```python
from build123d import *

# Parameters (mm, degrees)
SKETCH2_R           = 7.25
SKETCH2_R_2         = 2.25
SKETCH2_W           = 22
SKETCH2_H           = 44
BOSS_EXTRUDE1_DEPTH = 6
CUT_EXTRUDE1_START  = -26
CUT_EXTRUDE1_DEPTH  = 26


with BuildPart() as part:
    # Sketch2 → Boss-Extrude1 (new body)
    with BuildSketch(Plane(origin=(0, 0, 0), x_dir=(1, 0, 0), z_dir=(0, 1, 0))):
        with BuildLine():
            Line((-16.25, 90), (-16.25, -90))
            ThreePointArc((-16.25, -90), (0, -106.25), (16.25, -90))
            Line((16.25, -90), (16.25, 90))
            ThreePointArc((16.25, 90), (0, 106.25), (-16.25, 90))
        make_face()
        with Locations(Location((0, 90, 0), (0, 0, 270))):
            Circle(SKETCH2_R, mode=Mode.SUBTRACT)
        with Locations(Location((0, -90, 0), (0, 0, 270))):
            Circle(SKETCH2_R, mode=Mode.SUBTRACT)
        with Locations(Location((8, 98, 0), (0, 0, 270))):
            Circle(SKETCH2_R_2, mode=Mode.SUBTRACT)
        with Locations(Location((-8, 98, 0), (0, 0, 270))):
            Circle(SKETCH2_R_2, mode=Mode.SUBTRACT)
        with Locations(Location((-8, 82, 0), (0, 0, 270))):
            Circle(SKETCH2_R_2, mode=Mode.SUBTRACT)
        with Locations(Location((8, 82, 0), (0, 0, 270))):
            Circle(SKETCH2_R_2, mode=Mode.SUBTRACT)
        with Locations(Location((8, -98, 0), (0, 0, 90))):
            Circle(SKETCH2_R_2, mode=Mode.SUBTRACT)
        with Locations(Location((8, -82, 0), (0, 0, 90))):
            Circle(SKETCH2_R_2, mode=Mode.SUBTRACT)
        with Locations(Location((-8, -82, 0), (0, 0, 90))):
            Circle(SKETCH2_R_2, mode=Mode.SUBTRACT)
        with Locations(Location((-8, -98, 0), (0, 0, 90))):
            Circle(SKETCH2_R_2, mode=Mode.SUBTRACT)
        with Locations(Location((-5, 63.652785483, 0), (0, 0, 270))):
            Circle(SKETCH2_R_2, mode=Mode.SUBTRACT)
        with Locations(Location((5, 63.652785483, 0), (0, 0, 270))):
            Circle(SKETCH2_R_2, mode=Mode.SUBTRACT)
        with Locations(Location((-5, 14.152785483, 0), (0, 0, 270))):
            Circle(SKETCH2_R_2, mode=Mode.SUBTRACT)
        with Locations(Location((5, 14.152785483, 0), (0, 0, 270))):
            Circle(SKETCH2_R_2, mode=Mode.SUBTRACT)
        with Locations(Location((0, -36.453, 0), (0, 0, 270))):
            Circle(SKETCH2_R_2, mode=Mode.SUBTRACT)
        with Locations((0, 38.902785483)):
            Rectangle(SKETCH2_W, SKETCH2_H, mode=Mode.SUBTRACT)
    extrude(amount=BOSS_EXTRUDE1_DEPTH)

    # Sketch3 → Cut-Extrude1 (cut)
    with BuildSketch(Plane(origin=(0, 6, 0), x_dir=(1, 0, 0), z_dir=(0, 1, 0)).offset(CUT_EXTRUDE1_START)):
        with BuildLine():
            ThreePointArc((-2, -31.59887804), (-3.249097876, -32.329183443), (-4.25140088, -33.372725571))
            Line((-4.25140088, -33.372725571), (-12.25, -25.374126452))
            Line((-12.25, -25.374126452), (-12.25, 4.324358358))
            Line((-12.25, 4.324358358), (-2, -5.925641642))
            Line((-2, -5.925641642), (-2, -31.59887804))
        make_face()
        with BuildLine():
            ThreePointArc((4.25140088, -33.372725571), (3.249097876, -32.329183443), (2, -31.59887804))
            Line((2, -31.59887804), (2, -5.925641642))
            Line((2, -5.925641642), (12.25, 4.324358358))
            Line((12.25, 4.324358358), (12.25, -25.374126452))
            Line((12.25, -25.374126452), (4.25140088, -33.372725571))
        make_face()
        with BuildLine():
            ThreePointArc((-4.872043809, -38.408936892), (-4.138493695, -39.68338232), (-3.080274429, -40.70440088))
            Line((-3.080274429, -40.70440088), (-12.25, -49.874126451))
            Line((-12.25, -49.874126451), (-12.25, -31.030980701))
            Line((-12.25, -31.030980701), (-4.872043809, -38.408936892))
        make_face()
        with BuildLine():
            ThreePointArc((3.080274429, -40.70440088), (4.138493696, -39.68338232), (4.872043809, -38.408936892))
            Line((4.872043809, -38.408936892), (12.25, -31.030980701))
            Line((12.25, -31.030980701), (12.25, -49.874126451))
            Line((12.25, -49.874126451), (3.080274429, -40.70440088))
        make_face()
        with BuildLine():
            Line((-12.25, -55.530980701), (-12.25, -79.322921748))
            ThreePointArc((-12.25, -79.322921748), (-7.628207354, -75.651726495), (-2, -73.873546577))
            Line((-2, -73.873546577), (-2, -45.280980701))
            Line((-2, -45.280980701), (-12.25, -55.530980701))
        make_face()
        with BuildLine():
            ThreePointArc((12.25, -79.322921748), (7.628207354, -75.651726495), (2, -73.873546577))
            Line((2, -73.873546577), (2, -45.280980701))
            Line((2, -45.280980701), (12.25, -55.530980701))
            Line((12.25, -55.530980701), (12.25, -79.322921748))
        make_face()
        Polygon((-4.268787392, 2), (-9.421572875, 7.152785483), (-2, 7.152785483), (-2, 2), align=None)
        Polygon((2, 2), (4.268787392, 2), (9.421572875, 7.152785483), (2, 7.152785483), align=None)
    extrude(amount=CUT_EXTRUDE1_DEPTH, mode=Mode.SUBTRACT)


solid = part.part
```
Can you work these out from the model? Positions are in its coordinate system, mm. A direction names the side the tool comes from. Coordinates: 2 decimals unless noted, no trailing zeros. Loops run counter-clockwise (first coordinate to the right, second up) from the corner with the lowest first, then second, coordinate; pieces in that order, holes last. Notation, with made-up numbers: (-34.5, 81) -> (3.5, 81) arc R20 ccw to (3.5, 93) -> close; hole circle Ø1 at (34.25, 14.25). An arc over 180 degrees is marked (long way). Answer as a JSON object with one key per item and string values.
1) Imagine slicing it at A-A (z = 18). Please give me the cut outline in (x, y), then the cut area to 3 significant figures.
Results:
{"outline": "(-16.25, 0) -> (-12.25, 0) -> (-12.25, 6) -> (-16.25, 6) -> close; (-2, 0) -> (2, 0) -> (2, 6) -> (-2, 6) -> close; (12.25, 0) -> (16.25, 0) -> (16.25, 6) -> (12.25, 6) -> close", "area": "72.0 mm^2"}
2) If I drill on line 1 (X direction, y = 2.6, z = 62.5); line 2 (X direction, y = 4.8, z = 82); line 3 (Z direction, x = -1, y = 3.65), over which ranges is the centre line in solid material (lowest first)?
Results:
{"line 1": "x = -16.25 to -12.25, -2 to 2, 12.25 to 16.25", "line 2": "x = -16.25 to -10.25, -5.75 to 5.75, 10.25 to 16.25", "line 3": "z = -106.22 to -97.18, -82.82 to -60.9, -16.9 to 34.44, 38.47 to 82.82, 97.18 to 106.22"}
3) Imagine slicing it at C-C (y = 4.25). Count the separate pieces of the cut face and the enclosed holes in it, then the cut area to 3 significant figures.
Results:
{"separate pieces": "1", "enclosed holes": "24", "area": "3,830 mm^2"}
4) Imagine slicing it at B-B (z = -43.5). Please give me the cut outline in (x, y).
Results:
{"outline": "(-16.25, 0) -> (-11, 0) -> (-11, 6) -> (-16.25, 6) -> close; (11, 0) -> (16.25, 0) -> (16.25, 6) -> (11, 6) -> close"}
5) Imagine slicing it at D-D (x = 14.5). Please give me the cut outline in (y, z).
Results:
{"outline": "(0, -97.34) -> (6, -97.34) -> (6, 97.34) -> (0, 97.34) -> close"}
6) Thinking about a two-plate mould opening in Z: for faces 3 (the face through (-4.9, 3, -65.9)), 4 (the face through (-0.357, 2.958, 106.246)), 5 (the face through (0, 6, -1)), which applies, pulls with the +Z half, pulls with the -Z half, needs draft (parallel to the pull), parting line crosses it, or undercut?
Results:
{"face 3": "undercut", "face 4": "pulls with the +Z half", "face 5": "needs draft"}
7) For faces 1 (the face through (0.357, 2.958, -106.246)), 2 (the face through (11, 3, -39)), which set-ups out of +Z, -Z, +X, -X, +Y, -Y let a thin tool reach every point of the face, with its end or its side?
Results:
{"face 1": "-Z, +Y, -Y", "face 2": "+Y, -Y"}
8) For P1, Ø10, axis at x = 1.5, z = 8.5, coming from the -Y side; P2, Ø2, axis at x = -5.5, y = 4, coming from the -Z side; P3, Ø1.8, axis at x = 2, y = 4.5, coming from the -Z side; P4, Ø1, axis at x = 8, y = 4, coming from the -Z side, each with a flat end and sliding along its axis, tell me the tip position at first contact or that it passes through.
Results:
{"P1": "stops at y = 0", "P2": "stops at z = -105.61", "P3": "stops at z = -106.21", "P4": "stops at z = -104.42"}
